Verification items for the finished model (mm, model axes). Face numbers are marked on the shaded views. A direction names the side the tool comes from. Round coordinates to 2 decimals unless told otherwise and drop trailing zeros. Order: outer loops, then holes, each group sorted by start corner. A loop starts at its lowest first (then second) coordinate and runs counter-clockwise, first axis right, second up. Notation, with made-up numbers: (71, -32.75) -> (109, -32.75) arc R21 cw to (109, 6.25) -> close; hole circle Ø9 at (28.25, 63). An arc over 180 degrees is marked (long way). Answer in a Markdown table with one row per item. Add a question column.
Autodesk Inventor part; units mm, degrees
ref_plane "YZ Plane" through (0, 0, 0) normal (1, 0, 0) x (0, 1, 0)
ref_plane "XZ Plane" through (0, 0, 0) normal (0, 1, 0) x (-1, 0, 0)
ref_plane "XY Plane" through (0, 0, 0) normal (0, 0, 1) x (1, 0, 0)
sketch "Sketch1" plane through (0, 0, 0) normal (0, 0, 1) x (1, 0, 0)
  line L0 (-33.6993, 23.1981) -> (46.3007, 23.1981)
  line L1 (46.3007, 23.1981) -> (46.3007, -36.8019)
  line L2 (46.3007, -36.8019) -> (-33.6993, -36.8019)
  line L3 (-33.6993, -36.8019) -> (-33.6993, 23.1981)
  point P0 (0, 0)
  dimension "d0" = 80
  dimension "d1" = 60
extrude "Extrusion1" add sketch "Sketch1" along normal blind 50
sketch "Sketch2" plane through (0, 0, 50) normal (0, 0, 1) x (1, 0, 0)
  line L0 (-23.918, 27.4616) -> (-23.918, 18.4616)
  line L1 (-23.918, 18.4616) -> (-29.418, 18.4616)
  line L2 (-29.418, 18.4616) -> (-29.418, 8.4616)
  line L3 (-29.418, 8.4616) -> (-4.418, 8.4616)
  line L4 (-4.418, 8.4616) -> (-4.418, 18.4616)
  line L5 (-4.418, 18.4616) -> (-9.918, 18.4616)
  line L6 (-9.918, 18.4616) -> (-9.918, 27.4616)
  line L7 (-9.918, 27.4616) -> (-23.918, 27.4616)
  point P0 (0, 0)
  point P1 (-16.918, 27.4616)
  dimension "d4" = 14
  dimension "d5" = 10
  dimension "d6" = 25
  dimension "d7" = 9
  dimension "d8" = 7
  dimension "d9" = 12.5
extrude "Extrusion2" cut sketch "Sketch2" against normal blind 50
sketch "Sketch3" plane through (0, 0, 50) normal (0, 0, 1) x (1, 0, 0)
  line L0 (27.8246, 24.0009) -> (34.8246, 24.0009)
  line L1 (34.8246, 24.0009) -> (34.8246, 20.4151)
  line L2 (34.8246, 20.4151) -> (36.2388, 19.0009)
  line L3 (36.2388, 19.0009) -> (34.8246, 17.5867)
  line L4 (34.8246, 17.5867) -> (33.4104, 19.0009)
  line L5 (33.4104, 19.0009) -> (27.8246, 19.0009)
  line L6 (27.8246, 24.0009) -> (27.8246, 19.0009) construction
  line L7 (27.8246, 24.0009) -> (20.8246, 24.0009)
  line L8 (20.8246, 24.0009) -> (20.8246, 20.4151)
  line L9 (20.8246, 20.4151) -> (19.4104, 19.0009)
  line L10 (19.4104, 19.0009) -> (20.8246, 17.5867)
  line L11 (20.8246, 17.5867) -> (22.2388, 19.0009)
  line L12 (22.2388, 19.0009) -> (27.8246, 19.0009)
  point P0 (0, 0)
  dimension "d12" = 2
  dimension "d13" = 7
  dimension "d14" = 5
  dimension "d15" = 135
  dimension "d16" = 2
extrude "Extrusion3" cut sketch "Sketch3" against normal blind 50
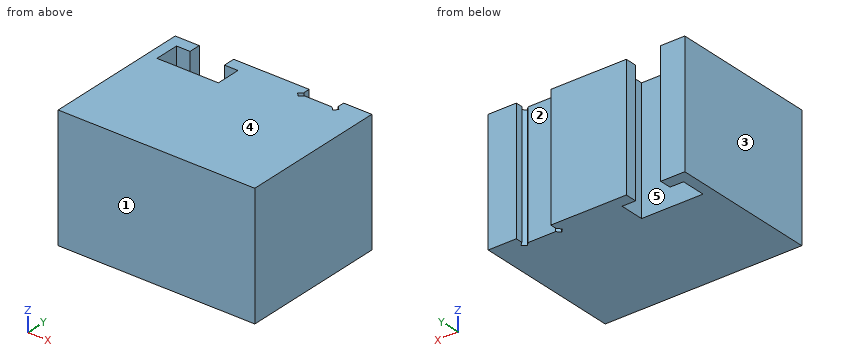
1) Tool access check on the marked faces 4 and 5. Record the directions out of +Z, -Z, +X, -X, +Y, -Y that give a thin tool (end or side, any length) a straight path to the whole face; none if there is none.
2) Cross-section at C-C, the plane z = 30.5. Record the boundary of the cut face in (x, y), and give its area (3 significant figures).
3) Draft check along X on the marked faces 1, 2 and 3. Enter one of: +X half, -X half, draft (parallel to the pull), parting line (faces both ways), or undercut.
4) Thickness scan on L1, parallel to X at y = 10, z = 27; L2, parallel to Y at x = 25, z = 32.5; L3, parallel to Y at x = -25, z = 21. Record the ranges inside material, lowest first. Write a range as [from, to].
5) Cross-section at A-A, the plane y = 13. Record the boundary of the cut face in (x, z).
6) Cross-section at B-B, the plane x = -25. Record the boundary of the cut face in (y, z), and give its area (3 significant figures).
7) Cross-section at D-D, the plane x = 31.5. Record the boundary of the cut face in (y, z).
Results below:
| question | item | result |
|---|---|---|
| 1 | face 4 | +Z, +X, -X, +Y, -Y |
| 1 | face 5 | +Z, -Z |
| 2 | outline | (-33.7, -36.8) -> (46.3, -36.8) -> (46.3, 23.2) -> (34.82, 23.2) -> (34.82, 20.42) -> (36.24, 19) -> (34.82, 17.59) -> (33.41, 19) -> (22.24, 19) -> (20.82, 17.59) -> (19.41, 19) -> (20.82, 20.42) -> (20.82, 23.2) -> (-9.92, 23.2) -> (-9.92, 18.46) -> (-4.42, 18.46) -> (-4.42, 8.46) -> (-29.42, 8.46) -> (-29.42, 18.46) -> (-23.92, 18.46) -> (-23.92, 23.2) -> (-33.7, 23.2) -> close |
| 2 | area | 4,420 mm² |
| 3 | face 1 | draft |
| 3 | face 2 | undercut |
| 3 | face 3 | -X half |
| 4 | L1 | [-33.7, -29.42], [-4.42, 46.3] |
| 4 | L2 | [-36.8, 19] |
| 4 | L3 | [-36.8, 8.46], [18.46, 23.2] |
| 5 | outline | (-33.7, 0) -> (-29.42, 0) -> (-29.42, 50) -> (-33.7, 50) -> close; (-4.42, 0) -> (46.3, 0) -> (46.3, 50) -> (-4.42, 50) -> close |
| 6 | outline | (-36.8, 0) -> (8.46, 0) -> (8.46, 50) -> (-36.8, 50) -> close; (18.46, 0) -> (23.2, 0) -> (23.2, 50) -> (18.46, 50) -> close |
| 6 | area | 2,500 mm² |
| 7 | outline | (-36.8, 0) -> (19, 0) -> (19, 50) -> (-36.8, 50) -> close |
